Autodesk Inventor part; units mm, degrees
ref_plane "YZ Plane" through (0, 0, 0) normal (1, 0, 0) x (0, 1, 0)
ref_plane "XZ Plane" through (0, 0, 0) normal (0, 1, 0) x (-1, 0, 0)
ref_plane "XY Plane" through (0, 0, 0) normal (0, 0, 1) x (1, 0, 0)
sketch "Sketch1" plane through (0, 0, 0) normal (0, 1, 0) x (-1, 0, 0)
  line L0 (-15.05, 18) -> (15.05, 18)
  line L1 (18, 15.05) -> (18, -15.05)
  line L2 (15.05, -18) -> (-15.05, -18)
  line L3 (-18, -15.05) -> (-18, 15.05)
  line L4 (-18, 18) -> (18, -18) construction
  line L5 (18, 18) -> (-18, -18) construction
  circle A0 centre (15.05, 15.05) radius 2
  circle A1 centre (-15.05, 15.05) radius 2
  circle A2 centre (-15.05, -15.05) radius 2
  circle A3 centre (15.05, -15.05) radius 2
  arc A4 (18, 15.05) -> (15.05, 18) centre (15.05, 15.05) ccw
  arc A5 (15.05, -18) -> (18, -15.05) centre (15.05, -15.05) ccw
  arc A6 (-18, -15.05) -> (-15.05, -18) centre (-15.05, -15.05) ccw
  arc A7 (-15.05, 18) -> (-18, 15.05) centre (-15.05, 15.05) ccw
  point P0 (0, 0)
  dimension "d0" = 36
  dimension "d1" = 36
  dimension "d2" = 4
  dimension "d3" = 15.05
  dimension "d6" = 360
  dimension "d8" = 2.95
extrude "Extrusion1" add sketch "Sketch1" along normal blind 15
properties part number "FC"
For this review, take the finished solid that the model builds, in its own axes (mm). Coordinates: 2 decimals unless noted, no trailing zeros. Write each loop counter-clockwise with the first axis right and the second up, starting at its lowest first coordinate (ties: lowest second). Pieces come first, ordered by that corner, then holes. Notation, with made-up numbers: (48, 84.25) -> (57, 84.25) arc R25 cw to (57, 100.25) -> close; hole circle Ø2 at (60.5, 53.25). An arc over 180 degrees is marked (long way). Put each result on its own line as item: value.
Q1. Take a section at C-C, the plane x = 15.5. State the section outline as (y, z) points, then the cut area to 3 significant figures.
From the geometry:
outline: (0, -17.97) -> (15, -17.97) -> (15, -17) -> (0, -17) -> close; (0, -13.1) -> (15, -13.1) -> (15, 13.1) -> (0, 13.1) -> close; (0, 17) -> (15, 17) -> (15, 17.97) -> (0, 17.97) -> close
area: 422 mm2
Q2. Wall thickness on L1, parallel to Z at x = -15.05, y = 8.25: over which ranges is the line inside the solid? List them lowest first.
From the geometry:
L1: z = -18 to -17.05, -13.05 to 13.05, 17.05 to 18
Q3. Take a section at B-B, the plane x = -16. State the section outline as (y, z) points, then the cut area to 3 significant figures.
From the geometry:
outline: (0, -17.84) -> (15, -17.84) -> (15, -16.81) -> (0, -16.81) -> close; (0, -13.29) -> (15, -13.29) -> (15, 13.29) -> (0, 13.29) -> close; (0, 16.81) -> (15, 16.81) -> (15, 17.84) -> (0, 17.84) -> close
area: 430 mm2
Q4. Take a section at A-A, the plane y = 8.75. State the section outline as (x, z) points.
From the geometry:
outline: (-18, -15.05) arc R2.95 ccw to (-15.05, -18) -> (15.05, -18) arc R2.95 ccw to (18, -15.05) -> (18, 15.05) arc R2.95 ccw to (15.05, 18) -> (-15.05, 18) arc R2.95 ccw to (-18, 15.05) -> close; hole circle Ø4 at (-15.05, -15.05); hole circle Ø4 at (-15.05, 15.05); hole circle Ø4 at (15.05, -15.05); hole circle Ø4 at (15.05, 15.05)
Q5. The part is to be moulded in two halves that separate along Z. For faces 1 (the flat face through (0, 7, -18)), 2 (the cylindrical face through (15.5, 7.4, -13.1)), 3 (the cylindrical face through (17.16, 7.4, 17.11)), say which applies: +Z half, -Z half, draft (parallel to the pull), parting line (faces both ways), or undercut.
From the geometry:
face 1: -Z half
face 2: undercut
face 3: +Z half
